Verification items for the finished model (mm, model axes). Face numbers are marked on the shaded views. A direction names the side the tool comes from. Coordinates: 2 decimals unless noted, no trailing zeros. Order: outer loops, then holes, each group sorted by start corner. A loop starts at its lowest first (then second) coordinate and runs counter-clockwise, first axis right, second up. Notation, with made-up numbers: (41, 79.5) - (79, 79.5) arc R31 cw to (79, 103.5) - close; hole circle Ø2 at (-27.75, 6.5). An arc over 180 degrees is marked (long way). One line per question, with ' | ' between items. Start each with the question number.
from build123d import *

# Parameters (mm, degrees)
SKETCH_W     = 701
SKETCH_H     = 300
PAD_DEPTH    = 179
SKETCH001_W  = 82.25
SKETCH001_H  = 214.5
PAD001_DEPTH = 67
SKETCH002_R  = 12.5
PAD002_DEPTH = 20
SKETCH003_R  = 12.5
PAD003_DEPTH = 20


with BuildPart() as part:
    # Sketch → Pad (new body)
    with BuildSketch(Plane.XY):
        Rectangle(SKETCH_W, SKETCH_H)
    extrude(amount=PAD_DEPTH)

    # Sketch001 → Pad001 (join)
    with BuildSketch(Plane.XY.offset(85)):
        with Locations((391.625, -0.5)):
            Rectangle(SKETCH001_W, SKETCH001_H)
    extrude(amount=PAD001_DEPTH)

    # Sketch002 → Pad002 (join)
    with BuildSketch(Plane.YZ.offset(432.75)):
        with Locations((-54, 125)):
            Circle(SKETCH002_R)
        with Locations((-27, 125)):
            Circle(SKETCH002_R)
    extrude(amount=PAD002_DEPTH)

    # Sketch003 → Pad003 (join)
    with BuildSketch(Plane.XZ.offset(107.75)):
        with Locations((367.5, 125)):
            Circle(SKETCH003_R)
    extrude(amount=PAD003_DEPTH)


solid = part.part
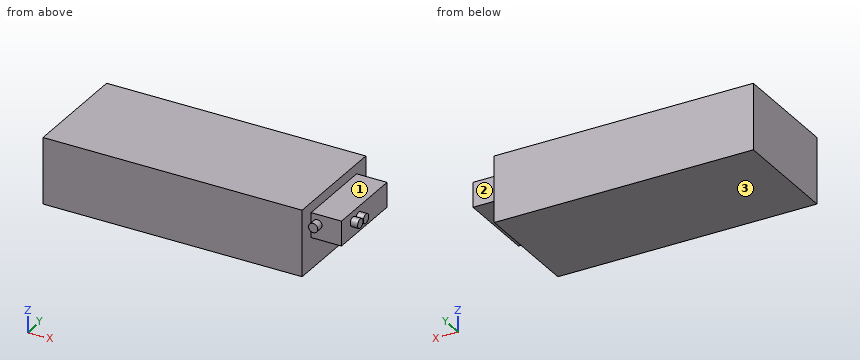
Item 1: Gauge pin test, flat ends, axial feed: pin 1 (1.5 mm diameter, centred on y = 104.5, z = 124.5, fed in from +X); pin 2 (1 mm diameter, centred on y = 119, z = 29, fed in from +X). Record the tip position at first contact, or that the pin passes through.
Item 2: Section check D-D (y = 18.5). Record the cut outline in (x, z), then the cut area to 3 significant figures.
Item 3: Set-up check for the marked faces 1, 2 and 3: record each of +Z, -Z, +X, -X, +Y, -Y from which the full face is reachable in a straight line by a thin tool's end or side.
Item 4: Section check B-B (x = 367.5). Record the cut outline in (y, z), then the cut area to 3 significant figures.
Item 5: Section check A-A (z = 125). Record the cut outline in (x, y), then the cut area to 3 significant figures.
Item 6: Thickness scan on probe 1 along X at (y, z) = (-21.5, 155.5); probe 2 along X at (y, z) = (15.5, 123); probe 3 along Z at (x, y) = (367.5, -118.5). Record the ranges inside material, lowest first. Write a range as from..to.
Item 7: Section check C-C (y = -54). Record the cut outline in (x, z), then the cut area to 3 significant figures.
Completed:
1) pin 1: stops at x = 432.75 | pin 2: stops at x = 350.5
2) outline: (-350.5, 0) - (350.5, 0) - (350.5, 85) - (432.75, 85) - (432.75, 152) - (350.5, 152) - (350.5, 179) - (-350.5, 179) - close | area: 131,000 mm^2
3) face 1: +Z, +X, +Y, -Y | face 2: +Z, -Z, +X, +Y | face 3: -Z, +X, -X, +Y, -Y
4) outline: (-127.75, 112.5) - (-107.75, 112.5) - (-107.75, 85) - (106.75, 85) - (106.75, 152) - (-107.75, 152) - (-107.75, 137.5) - (-127.75, 137.5) - close | area: 14,900 mm^2
5) outline: (-350.5, -150) - (350.5, -150) - (350.5, -107.75) - (355, -107.75) - (355, -127.75) - (380, -127.75) - (380, -107.75) - (432.75, -107.75) - (432.75, -66.5) - (452.75, -66.5) - (452.75, -41.5) - (432.75, -41.5) - (432.75, -39.5) - (452.75, -39.5) - (452.75, -14.5) - (432.75, -14.5) - (432.75, 106.75) - (350.5, 106.75) - (350.5, 150) - (-350.5, 150) - close | area: 229,000 mm^2
6) probe 1: x = -350.5..350.5 | probe 2: x = -350.5..432.75 | probe 3: z = 112.5..137.5
7) outline: (-350.5, 0) - (350.5, 0) - (350.5, 85) - (432.75, 85) - (432.75, 112.5) - (452.75, 112.5) - (452.75, 137.5) - (432.75, 137.5) - (432.75, 152) - (350.5, 152) - (350.5, 179) - (-350.5, 179) - close | area: 131,000 mm^2
